For this review, take the finished solid that the model builds, in its own axes (mm). A direction names the side the tool comes from. Coordinates: 2 decimals unless noted, no trailing zeros. Loops run counter-clockwise (first coordinate to the right, second up) from the corner with the lowest first, then second, coordinate; pieces in that order, holes last. Notation, with made-up numbers: (41, 83.25) -> (73, 83.25) arc R19 ccw to (73, 111.25) -> close; hole circle Ø6 at (42.25, 24). An arc over 180 degrees is marked (long way). Use a Markdown table: item, result.
from build123d import *

# Parameters (mm, degrees)
SKETCH1_R            = 140
SKETCH1_R_2          = 97
BOSS_EXTRUDE7_DEPTH  = 225
SKETCH1_5_R          = 23.5
BOSS_EXTRUDE9_DEPTH  = 32
SKETCH2_R            = 100
SKETCH2_R_2          = 12
SKETCH2_R_3          = 50
BOSS_EXTRUDE11_DEPTH = 61
SKETCH2_4_R          = 12
CUT_EXTRUDE1_DEPTH   = 15
SKETCH2_5_R          = 25
CUT_EXTRUDE2_DEPTH   = 547


with BuildPart() as part:
    # Sketch1 → Boss-Extrude7 (new body)
    with BuildSketch(Plane(origin=(0, 0, 0), x_dir=(1, 0, 0), z_dir=(0, 1, 0))):
        with Locations(Location((0, 0, 0), (0, 0, 270))):
            Circle(SKETCH1_R)
        with Locations(Location((0, 0, 0), (0, 0, 270))):
            Circle(SKETCH1_R_2, mode=Mode.SUBTRACT)
    extrude(amount=BOSS_EXTRUDE7_DEPTH)

    # Sketch1_5 → Boss-Extrude9 (add)
    with BuildSketch(Plane(origin=(0, 0, 0), x_dir=(1, 0, 0), z_dir=(0, 1, 0))):
        with BuildLine():
            Line((176.554445662, -44.198729811), (138.247516529, -22.082213964))
            ThreePointArc((138.247516529, -22.082213964), (121.24355653, -70), (88.247516529, -108.684754342))
            Line((88.247516529, -108.684754342), (126.554445662, -130.801270189))
            ThreePointArc((126.554445662, -130.801270189), (194.855715852, -112.5), (176.554445662, -44.198729811))
        make_face()
        with Locations(Location((151.554445662, -87.5, 0), (0, 0, 270))):
            Circle(SKETCH1_5_R, mode=Mode.SUBTRACT)
        with BuildLine():
            Line((50, 130.766968306), (50, 175))
            ThreePointArc((50, 175), (0, 225), (-50, 175))
            Line((-50, 175), (-50, 130.766968306))
            ThreePointArc((-50, 130.766968306), (0, 140), (50, 130.766968306))
        make_face()
        with Locations(Location((0, 175, 0), (0, 0, 270))):
            Circle(SKETCH1_5_R, mode=Mode.SUBTRACT)
        with BuildLine():
            ThreePointArc((-88.247516529, -108.684754342), (-121.24355653, -70), (-138.247516529, -22.082213964))
            Line((-138.247516529, -22.082213964), (-176.554445662, -44.198729811))
            ThreePointArc((-176.554445662, -44.198729811), (-194.855715851, -112.5), (-126.554445662, -130.801270189))
            Line((-126.554445662, -130.801270189), (-88.247516529, -108.684754342))
        make_face()
        with Locations(Location((-151.554445662, -87.5, 0), (0, 0, 270))):
            Circle(SKETCH1_5_R, mode=Mode.SUBTRACT)
    boss_extrude9 = extrude(amount=BOSS_EXTRUDE9_DEPTH)

    # Mirror1: Boss-Extrude9 across plane
    add(boss_extrude9.mirror(Plane.ZX.offset(112.5)))

    # Sketch2 → Boss-Extrude11 (add)
    with BuildSketch(Plane.XY.offset(165)):
        with Locations((0, 112.5)):
            Circle(SKETCH2_R)
        with Locations((-64.951905284, 75)):
            Circle(SKETCH2_R_2, mode=Mode.SUBTRACT)
        with Locations((64.951905284, 75)):
            Circle(SKETCH2_R_2, mode=Mode.SUBTRACT)
        with Locations((0, 187.5)):
            Circle(SKETCH2_R_2, mode=Mode.SUBTRACT)
        with Locations((0, 112.5)):
            Circle(SKETCH2_R_3, mode=Mode.SUBTRACT)
        with Locations((64.951905284, 75)):
            Circle(SKETCH2_R_2)
        with Locations((-64.951905284, 75)):
            Circle(SKETCH2_R_2)
        with Locations((0, 187.5)):
            Circle(SKETCH2_R_2)
    extrude(amount=-BOSS_EXTRUDE11_DEPTH)

    # Sketch2_4 → Cut-Extrude1 (cut)
    with BuildSketch(Plane.XY.offset(165)):
        with Locations((0, 187.5)):
            Circle(SKETCH2_4_R)
        with Locations((64.951905284, 75)):
            Circle(SKETCH2_4_R)
        with Locations((-64.951905284, 75)):
            Circle(SKETCH2_4_R)
    extrude(amount=-CUT_EXTRUDE1_DEPTH, mode=Mode.SUBTRACT)

    # Sketch2_5 → Cut-Extrude2 (cut)
    with BuildSketch(Plane.XY.offset(165)):
        with Locations((0, 112.5)):
            Circle(SKETCH2_5_R)
    extrude(amount=-CUT_EXTRUDE2_DEPTH, mode=Mode.SUBTRACT)


solid = part.part
(1) For pin 1 Ø21.5 at (x, y) = (-64.95, 75) entering from +Z; pin 2 Ø1 at (x, y) = (24.5, 41) entering from -Z; pin 3 Ø4 at (y, z) = (123.5, -63) entering from +X, all flat-tipped, find the tip position at first contact; note any pin that passes through.
Found:
| item | result |
|---|---|
| pin 1 | stops at z = 150 |
| pin 2 | stops at z = -137.93 |
| pin 3 | stops at x = 126.01 |
(2) Take a section at A-A on x = 36. Write out the cut boundary in (y, z), plus the area to 3 significant figures.
Found:
| item | result |
|---|---|
| outline | (0, -209.7) -> (32, -209.7) -> (32, -135.29) -> (193, -135.29) -> (193, -209.7) -> (225, -209.7) -> (225, -90.07) -> (0, -90.07) -> close; (0, 90.07) -> (225, 90.07) -> (225, 135.29) -> (205.8, 135.29) -> (205.8, 165) -> (147.2, 165) -> (147.2, 135.29) -> (77.8, 135.29) -> (77.8, 165) -> (19.2, 165) -> (19.2, 135.29) -> (0, 135.29) -> close |
| area | 28,600 mm^2 |
(3) Take a section at C-C on y = 153. Write out the cut boundary in (x, z), plus the area to 3 significant figures.
Found:
| item | result |
|---|---|
| outline | (-91.43, 106.02) arc R140 ccw (long way) to (91.43, 106.02) -> (91.43, 165) -> (29.32, 165) -> (29.32, 136.9) arc R140 ccw to (-29.32, 136.9) -> (-29.32, 165) -> (-91.43, 165) -> close; hole circle Ø194 at (0, 0) |
| area | 37,000 mm^2 |
(4) Take a section at B-B on z = -40.5. Write out the cut boundary in (x, y), plus the area to 3 significant figures.
Found:
| item | result |
|---|---|
| outline | (-134.01, 0) -> (-88.14, 0) -> (-88.14, 225) -> (-134.01, 225) -> close; (88.14, 0) -> (134.01, 0) -> (134.01, 225) -> (88.14, 225) -> close |
| area | 20,600 mm^2 |
(5) Take a section at D-D on x = -161.5. Write out the cut boundary in (y, z).
Found:
| item | result |
|---|---|
| outline | (0, 35.51) -> (32, 35.51) -> (32, 66.21) -> (0, 66.21) -> close; (0, 108.79) -> (32, 108.79) -> (32, 136.5) -> (0, 136.5) -> close; (193, 35.51) -> (225, 35.51) -> (225, 66.21) -> (193, 66.21) -> close; (193, 108.79) -> (225, 108.79) -> (225, 136.5) -> (193, 136.5) -> close |
(6) Mouldability with a two-part tool opening along X and no side actions: class faces 1 (the face through (169, 32, 105)), 2 (the face through (157.669, 209.224, 33.295)), 3 (the face through (1.033, 209.224, -198.477)) as pulls with the +X half, pulls with the -X half, needs draft (parallel to the pull), parting line crosses it, or undercut.
Found:
| item | result |
|---|---|
| face 1 | needs draft |
| face 2 | pulls with the +X half |
| face 3 | undercut |
(7) For faces 4 (the face through (107.133, 15.776, 119.588)), 5 (the face through (50, 209, -153)), 6 (the face through (55.43, 67.7, 157.6)), list the 3-axis set-ups (+Z, -Z, +X, -X, +Y, -Y) from which the entire face can be reached by the end or side of a thin tool; tool diameter is ignored.
Found:
| item | result |
|---|---|
| face 4 | +Z, -Y |
| face 5 | -Z, +X, +Y, -Y |
| face 6 | +Z |
(8) For line 1 along Y through (x, z) = (0, 145.5); line 2 along X through (y, z) = (206, 87); line 3 along Y through (x, z) = (178, 118), list the stretches that pass through material, from the lowest coordinate up.
Found:
| item | result |
|---|---|
| line 1 | y = 12.5 to 62.5, 162.5 to 212.5 |
| line 2 | x = -201.55 to -175.05, -128.06 to -42.9, 42.9 to 128.06, 175.05 to 201.55 |
| line 3 | y = 0 to 32, 193 to 225 |
